Geometry check sheet. Reference: the model listing, model coordinates, mm. Round coordinates to 2 decimals unless told otherwise and drop trailing zeros. Loops run counter-clockwise (first coordinate to the right, second up) from the corner with the lowest first, then second, coordinate; pieces in that order, holes last. Notation, with made-up numbers: (-26.75, -35) -> (30.25, -35) arc R13 cw to (30.25, -22) -> close; hole circle Ø1 at (-22.5, 75.25). An arc over 180 degrees is marked (long way). Use a Markdown table: item, result. Add a question column.
Q1. Sectioned sample at C-C, the plane y = 179. Enter the section's corners in (x, z), then the cut area to 3 significant figures.
Q2. Gauge pin test, flat end, axial feed: P1, Ø1, axis at x = -1, y = 226, coming from the +Z side. Record the tip position at first contact, or that the pin passes through.
Q3. Sectioned sample at D-D, the plane y = 111.5. Enter the section's corners in (x, z), then the cut area to 3 significant figures.
Q4. Material ranges on L1, parallel to Y at x = -0.5, z = 65; L2, parallel to Z at x = -1.1, y = 172; L3, parallel to Z at x = 0.05, y = 89.5, recorded low to high.
Q5. Sectioned sample at B-B, the plane x = 0.35. Enter the section's corners in (y, z), then the cut area to 3 significant figures.
Q6. Sectioned sample at A-A, the plane z = 189. Enter the section's corners in (x, y).
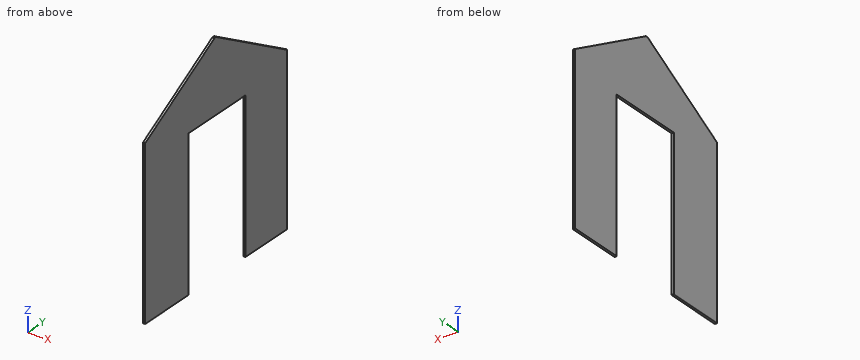
```python
from build123d import *

# Parameters (mm, degrees)
BOX013_W               = 10
BOX013_H               = 140
BOX013_DEPTH           = 270
BOX009_W               = 18
BOX009_H               = 200
BOX009_DEPTH           = 87
BOX009_PLACEMENT_ANGLE = 30
BOX008_W               = 18
BOX008_H               = 200
BOX008_DEPTH           = 87
BOX008_PLACEMENT_ANGLE = 30
BOX007_W               = 348
BOX007_H               = 4
BOX007_DEPTH           = 400


with BuildPart() as door:
    # Box013 → Box013 (new body)
    with BuildSketch(Plane(origin=(-5, 106, 0), x_dir=(1, 0, 0), z_dir=(0, 0, 1))):
        with Locations((5, 70)):
            Rectangle(BOX013_W, BOX013_H)
    extrude(amount=BOX013_DEPTH)


with BuildPart() as box009:
    # Box009 → Box009 (new body)
    with BuildSketch(Plane.XY):
        with Locations((9, 100)):
            Rectangle(BOX009_W, BOX009_H)
    extrude(amount=BOX009_DEPTH)


with BuildPart() as box009_1:
    # Box009 placement: moved
    add(box009.part.moved(Location((598, 174.528857, 399.719854))).rotate(Axis((598, 174.528857, 399.719854), (-1, 0, 0)), BOX009_PLACEMENT_ANGLE))


with BuildPart() as box008:
    # Box008 → Box008 (new body)
    with BuildSketch(Plane.XY):
        with Locations((9, 100)):
            Rectangle(BOX008_W, BOX008_H)
    extrude(amount=BOX008_DEPTH)


with BuildPart() as box008_1:
    # Box008 placement: moved
    add(box008.part.moved(Location((598, -0.25833, 301.447441))).rotate(Axis((598, -0.25833, 301.447441), (1, 0, 0)), BOX008_PLACEMENT_ANGLE))


with BuildPart() as cut004:
    # Box007 → Box007 (new body)
    with BuildSketch(Plane(origin=(605, 0, 0), x_dir=(0, 1, 0), z_dir=(0, 0, 1))):
        with Locations((174, 2)):
            Rectangle(BOX007_W, BOX007_H)
    extrude(amount=BOX007_DEPTH)

    # Cut002: cut Box008
    add(box008_1.part, mode=Mode.SUBTRACT)

    # Cut003: cut Box009
    add(box009_1.part, mode=Mode.SUBTRACT)


with BuildPart() as cut004_1:
    # Cut003 placement: moved
    add(cut004.part.moved(Location((-604, 0, 0))))

    # Cut004: cut Door
    add(door.part, mode=Mode.SUBTRACT)


solid = cut004_1.part
```
Values:
| question | item | result |
|---|---|---|
| 1 | outline | (-3, 270) -> (1, 270) -> (1, 397.14) -> (-3, 397.14) -> close |
| 1 | area | 509 mm^2 |
| 2 | P1 | z = 370.29 |
| 3 | outline | (-3, 270) -> (1, 270) -> (1, 365.97) -> (-3, 365.97) -> close |
| 3 | area | 384 mm^2 |
| 4 | L1 | 0 to 106, 246 to 348 |
| 4 | L2 | 270 to 400 |
| 4 | L3 | 0 to 353.27 |
| 5 | outline | (0, 0) -> (106, 0) -> (106, 270) -> (246, 270) -> (246, 0) -> (348, 0) -> (348, 300.18) -> (347.73, 299.72) -> (174.53, 399.72) -> (174.69, 400) -> (170.44, 400) -> (0, 301.6) -> close |
| 5 | area | 84,300 mm^2 |
| 6 | outline | (-3, 0) -> (1, 0) -> (1, 106) -> (-3, 106) -> close; (-3, 246) -> (1, 246) -> (1, 348) -> (-3, 348) -> close |
